Here's how the part is built. I have some questions about the finished solid (model axes, mm). A direction names the side the tool comes from. Round coordinates to 2 decimals unless told otherwise and drop trailing zeros. Write each loop counter-clockwise with the first axis right and the second up, starting at its lowest first coordinate (ties: lowest second). Pieces come first, ordered by that corner, then holes. Notation, with made-up numbers: (6.25, 57) - (33.25, 57) arc R13 ccw to (33.25, 80) - close; hole circle Ø1 at (-35, 7.25). An arc over 180 degrees is marked (long way). Write item = value, one per line. Start each with the question number.
Item 1: If we section it at D-D (x = 3.5): Please give me the cut outline in (y, z), and give its area (3 significant figures).
Item 2: If we section it at C-C (y = 19): Please give me the cut outline in (x, z).
Item 3: For P1, Ø5, axis at y = 19, z = -10, coming from the +X side; P2, Ø1, axis at x = 1, z = -0.5, coming from the +Y side; P3, Ø1.3, axis at x = 4.5, z = -7.5, coming from the -Y side, each with a flat end and sliding along its axis, tell me the tip position at first contact or that it passes through.
Item 4: Which directions (+Z, -Z, +X, -X, +Y, -Y) give clear straight access to the entire face, cutting with the end or side of a thin tool? Please do faces 4 (the face through (-2, 15, -8.5)), 5 (the face through (3, 7, 8)), 6 (the face through (-2, 20, 0)), 7 (the face through (0, 12, 0)).
Item 5: If we section it at B-B (z = -8.1): Please give me the cut outline in (x, y).
Item 6: If I drill on line 1 along Z through (x, y) = (3.5, 3.45); line 2 along X through (y, z) = (4.7, 8.1); line 3 along Y through (x, z) = (-1.9, 10), over which ranges is the centre line in solid material (lowest first)? Write a range as [from, to].
Item 7: Thinking about a two-plate mould opening in Z: for faces 1 (the face through (-1, 8, 12.5)), 2 (the face through (3, 8, 0)), 3 (the face through (-2, 15, 8.5)), which applies, pulls with the +Z half, pulls with the -Z half, needs draft (parallel to the pull), parting line crosses it, or undercut?
Item 8: If we section it at A-A (y = 16.75): Please give me the cut outline in (x, z).
Autodesk Inventor part; units mm, degrees
ref_plane "РабПлоскость7" through (-3, 0, 6) normal (-1, 0, 0) x (0, 0, 1)
ref_plane "YZ Plane" through (0, 0, 0) normal (1, 0, 0) x (0, 1, 0)
ref_plane "XZ Plane" through (0, 0, 0) normal (0, 1, 0) x (-1, 0, 0)
ref_plane "РабПлоскость7" through (-3, 0, 6) normal (-1, 0, 0) x (0, 0, 1)
sketch "Эскиз3" plane through (-3, 0, 6) normal (-1, 0, 0) x (0, 0, 1)
  line L0 (0, 0) -> (-12, 0) construction
  line L1 (0, 0) -> (0, 23.3031) construction
  line L2 (3, 0) -> (3, 3) construction
  circle A0 centre (-16, 19) radius 1.5
  circle A1 centre (4, 19) radius 1.5
  line L3 (-17.5, 19) -> (-18.5, 19)
  line L4 (-16, 20.5) -> (-16, 21.5)
  line L5 (-18.5, 21.5) -> (6.5, 21.5)
  line L6 (6.5, 21.5) -> (6.5, 13)
  line L7 (-18.5, 13) -> (-18.5, 21.5)
  line L8 (-18.5, 8) -> (-18.5, 13)
  line L9 (6.5, 8) -> (6.5, 13)
  line L10 (2.5, 17.5) -> (-14.5, 17.5)
  line L11 (-14.5, 17.5) -> (-14.5, 13)
  line L12 (-14.5, 13) -> (2.5, 13)
  line L13 (2.5, 13) -> (2.5, 17.5)
  line L14 (-3, 13) -> (-3, 8)
  line L15 (-9, 3) -> (-9, 13)
  line L16 (6.5, 8) -> (-4, 8)
  line L17 (-4, 8) -> (-4, 13)
  line L18 (-18.5, 8) -> (-8, 8)
  line L19 (-8, 8) -> (-8, 13)
  line L20 (-8, 8) -> (-4, 8)
  point P0 (-6, 0)
  point P1 (-9, 8)
  point P2 (-9, 8)
  dimension "d55" = 3
  dimension "d56" = 3
  dimension "d57" = 1
  dimension "d58" = 1
  dimension "d59" = 25
  dimension "d68" = 10.5
  dimension "d69" = 10.5
extrude "Выдавливание10" add sketch "Эскиз3" against normal blind 3 contours A0 L4 L5 L6 L9 L16 L14 L12 L13 L10 L11 L15 L18 L8 L7 L3 | A0 L3 L7 L5 L4 | L15 L12 L19 L18 | L16 L17 L12 L14
extrude "Выдавливание12" add sketch "Эскиз3" against normal blind 3 contours L19 L12 L17 L20
sketch "Эскиз5" plane through (-3, 8, -12.5) normal (0, -1, 0) x (1, 0, 0)
  line L0 (7.899, 12.5) -> (3, 12.5) construction
  line L1 (0, 25) -> (10, 25)
  line L2 (10, 25) -> (10, 0)
  line L3 (10, 0) -> (0, 0)
  line L4 (0, 0) -> (0, 25)
  circle A0 centre (6.5, 4.4) radius 2.1
  line L5 (3, 25) -> (6.5, 25)
  line L6 (6.5, 25) -> (6.5, 0)
  circle A1 centre (6.5, 20.6) radius 2.1
  point P0 (8, 5.5)
  point P1 (6.5, 18.5)
  point P2 (6.5, 6.5)
  point P3 (6.5, 4.4)
  dimension "d94" = 10
  dimension "d95" = 25
  dimension "d96" = 4.2
  dimension "d102" = 3.5
extrude "Выдавливание13" [suppressed]
fillet "Сопряжение18" [suppressed]
fillet "Сопряжение19" radius 2 2 edges at (-1.5, 21.5, -12.5) (-1.5, 21.5, 12.5)
extrude "Выдавливание14" add sketch "Эскиз5" along normal blind 7
extrude "Выдавливание15" cut sketch "Эскиз5" against normal blind 6 from surface at 7 contours L6 A0 | A0 L6
fillet "Сопряжение20" radius 2 2 edges at (7, 4.5, -12.5) (7, 4.5, 12.5)
extrude "Выдавливание16" cut sketch "Эскиз5" against normal blind 6 from surface at 7 contours A1 L6 | L6 A1
sketch "Эскиз6" plane through (-3, 0, 6) normal (-1, 0, 0) x (0, 0, 1)
  point P0 (-6, 0)
sketch "Эскиз8" plane through (0, 0, 6) normal (1, 0, 0) x (0, 0, -1)
  circle A0 centre (-4, 19) radius 1.5 construction
  line L0 (-2.5, 19) -> (-1.5, 19) construction
  line L1 (-4.5, 21.5) -> (16.5, 21.5)
  line L2 (-2.5, 17.5) -> (14.5, 17.5)
  line L3 (-1.5, 21.5) -> (13.5, 21.5) construction
  line L4 (13.5, 21.5) -> (13.5, 17.5)
  line L5 (13.5, 17.5) -> (-1.5, 17.5) construction
  line L6 (-1.5, 17.5) -> (-1.5, 21.5)
  point P0 (6, 0)
  dimension "d105" = 1
  dimension "d106" = 15
extrude "Выдавливание17" cut sketch "Эскиз8" against normal blind 2
properties part number "крепл_ЛД"
Reply:
q1.outline = (1, -12.5) - (8, -12.5) - (8, 12.5) - (1, 12.5) - (1, 10.2) - (7, 10.2) - (7, 6) - (1, 6) - (1, -6) - (7, -6) - (7, -10.2) - (1, -10.2) - close
q1.area = 125 mm2
q2.outline = (-3, -12.5) - (0, -12.5) - (0, -11.5) - (-3, -11.5) - close; (-3, -8.5) - (0, -8.5) - (0, -7.5) - (-2, -7.5) - (-2, 7.5) - (0, 7.5) - (0, 8.5) - (-3, 8.5) - close; (-3, 11.5) - (0, 11.5) - (0, 12.5) - (-3, 12.5) - close
q3.P1 = 0
q3.P2 = 8
q3.P3 = 7
q4.face_4 = +X, -X
q4.face_5 = -Y
q4.face_6 = +X, +Y
q4.face_7 = +Z, -Z, +X, +Y
q5.outline = (-3, 1) - (1.4, 1) - (1.4, 7) - (5.6, 7) - (5.6, 1) - (7, 1) - (7, 8) - (0, 8) - (0, 13) - (-3, 13) - close; (-3, 17.5) - (0, 17.5) - (0, 21.5) - (-3, 21.5) - close
q6.line_1 = [-12.5, -10.2], [-6, 6], [10.2, 12.5]
q6.line_2 = [-3, 1.4], [5.6, 7]
q6.line_3 = [1, 17.5], [20.5, 21.5]
q7.face_1 = pulls with the +Z half
q7.face_2 = needs draft
q7.face_3 = undercut
q8.outline = (-3, -12.5) - (0, -12.5) - (0, -8.5) - (-3, -8.5) - close; (-3, 8.5) - (0, 8.5) - (0, 12.5) - (-3, 12.5) - close
